For this review, take the finished solid that the model builds, in its own axes (mm). Face numbers are marked on the shaded views. A direction names the side the tool comes from. Coordinates: 2 decimals unless noted, no trailing zeros. Loops run counter-clockwise (first coordinate to the right, second up) from the corner with the lowest first, then second, coordinate; pieces in that order, holes last.
1. Take a section at B-B, the plane x = 0.5. State the section outline as (y, z) points.
2. Clearance check with flat-ended pins moving along their axes: P1, Ø1, axis at x = -16.5, z = 1, coming from the -Y side; P2, Ø0.6, axis at x = -9, z = 1, coming from the -Y side; P3, Ø0.6, axis at y = -2.5, z = 1, coming from the -X side; P4, Ø5, axis at x = -8, y = 0, coming from the -Z side. State where each tip first meets the part, or that it passes through.
3. Machinability: for the marked faces 4, 5, 6 and 7, which of the approach directions +Z, -Z, +X, -X, +Y, -Y give a long, thin tool a straight path to every point of the face, cutting with its end or side? Answer none if there is none.
4. To check wall thickness, follow probe 1 along X at (y, z) = (0.75, 0.6); probe 2 along X at (y, z) = (-3.25, 1.4); probe 3 along X at (y, z) = (-5.5, 0.75). State the ranges of each line that lie inside material, in increasing order.
5. Take a section at D-D, the plane x = -8.25. State the section outline as (y, z) points, then the cut area to 3 significant figures.
6. Take a section at C-C, the plane z = 1.7. State the section outline as (x, y) points, then the cut area to 3 significant figures.
7. Take a section at A-A, the plane y = 0.5. State the section outline as (x, z) points, then the cut area to 3 significant figures.
8. Mouldability with a two-part tool opening along Y and no side actions: class the marked faces 1, 2 and 3 as pulls with the +Y half, pulls with the -Y half, needs draft (parallel to the pull), parting line crosses it, or undercut.
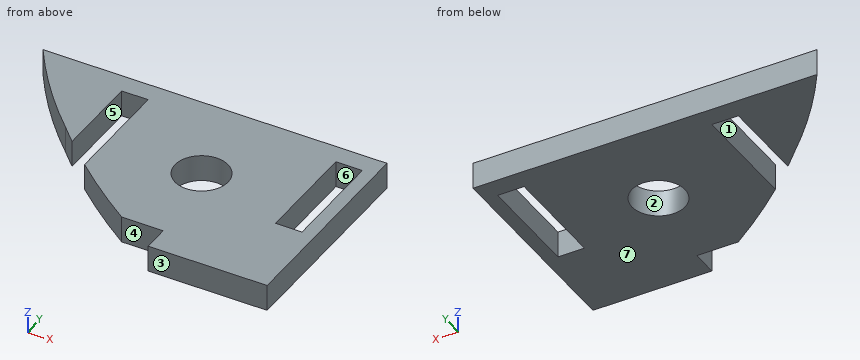
```python
from build123d import *

# Parameters (mm, degrees)
SKETCH1_R           = 2
SKETCH1_W           = 2
SKETCH1_H           = 8
BOSS_EXTRUDE1_DEPTH = 2


with BuildPart() as part:
    # Sketch1 → Boss-Extrude1 (new body)
    with BuildSketch(Plane.XY):
        with BuildLine():
            Line((-6.654132998, -12.706050279), (-6.654132998, -10.706050279))
            Line((-6.654132998, -10.706050279), (-9.783639909, -10.706050279))
            ThreePointArc((-9.783639909, -10.706050279), (-12.367491039, -8.806551261), (-14.831802528, -6.754344625))
            Line((-14.831802528, -6.754344625), (-14.831802528, 1.669576319))
            Line((-14.831802528, 1.669576319), (-16.831802528, 1.669576319))
            Line((-16.831802528, 1.669576319), (-16.831802528, -4.889537014))
            ThreePointArc((-16.831802528, -4.889537014), (-17.420540419, -4.302376557), (-18, -3.706057599))
            ThreePointArc((-18, -3.706057599), (-21.006837803, -0.430380182), (-23.616713146, 3.169576319))
            Line((-23.616713146, 3.169576319), (2.324507934, 3.169576319))
            Line((2.324507934, 3.169576319), (2.324507934, -12.706050279))
            Line((2.324507934, -12.706050279), (-6.654132998, -12.706050279))
        make_face()
        with Locations((-7.675492066, -3.830423681)):
            Circle(SKETCH1_R, mode=Mode.SUBTRACT)
        with Locations((0.324507934, -2.330423681)):
            Rectangle(SKETCH1_W, SKETCH1_H, mode=Mode.SUBTRACT)
    extrude(amount=BOSS_EXTRUDE1_DEPTH)


solid = part.part
```
Results list:
1. outline: (-12.71, 0) - (-6.33, 0) - (-6.33, 2) - (-12.71, 2) - close; (1.67, 0) - (3.17, 0) - (3.17, 2) - (1.67, 2) - close
2. P1: stops at y = -4.89
2. P2: stops at y = -10.71
2. P3: stops at x = -19.47
2. P4: stops at z = 0
3. face 4: +Z, -Z, -X, -Y
3. face 5: +Z, -Z, -Y
3. face 6: +Z, -Z
3. face 7: -Z, +X, -X, +Y, -Y
4. probe 1: x = -21.93 to -16.83, -14.83 to -0.68, 1.32 to 2.32
4. probe 2: x = -18.46 to -16.83, -14.83 to -9.59, -5.76 to -0.68, 1.32 to 2.32
4. probe 3: x = -14.83 to -8.78, -6.57 to -0.68, 1.32 to 2.32
5. outline: (-10.71, 0) - (-5.75, 0) - (-5.75, 2) - (-10.71, 2) - close; (-1.91, 0) - (3.17, 0) - (3.17, 2) - (-1.91, 2) - close
5. area: 20.1 mm2
6. outline: (-23.62, 3.17) arc R38.57 ccw to (-18, -3.71) arc R53.03 ccw to (-16.83, -4.89) - (-16.83, 1.67) - (-14.83, 1.67) - (-14.83, -6.75) arc R53.03 ccw to (-9.78, -10.71) - (-6.65, -10.71) - (-6.65, -12.71) - (2.32, -12.71) - (2.32, 3.17) - close; hole circle Ø4 at (-7.68, -3.83); hole (-0.68, -6.33) - (1.32, -6.33) - (1.32, 1.67) - (-0.68, 1.67) - close
6. area: 250 mm2
7. outline: (-21.74, 0) - (-16.83, 0) - (-16.83, 2) - (-21.74, 2) - close; (-14.83, 0) - (-0.68, 0) - (-0.68, 2) - (-14.83, 2) - close; (1.32, 0) - (2.32, 0) - (2.32, 2) - (1.32, 2) - close
7. area: 40.1 mm2
8. face 1: needs draft
8. face 2: undercut
8. face 3: pulls with the -Y half
